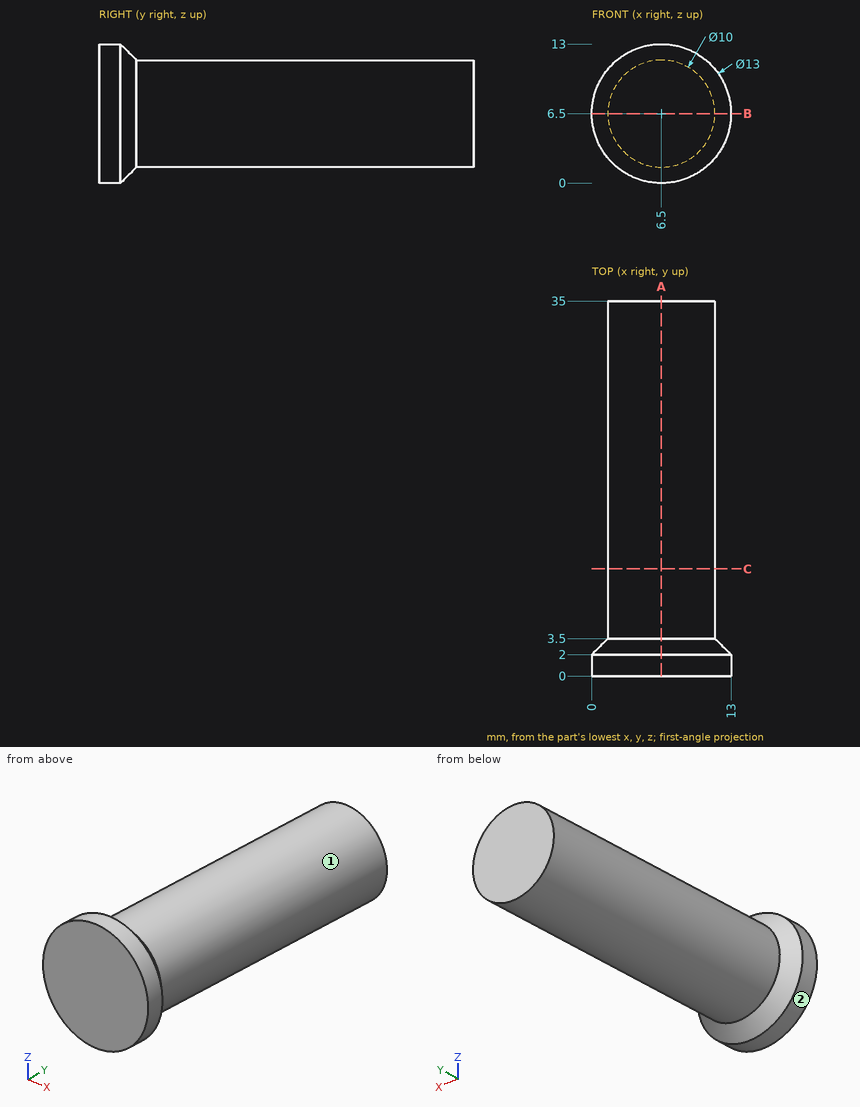
Geometry check sheet. Reference: drawing and pictorial views, mm from the part's lowest x, y, z. A direction names the side the tool comes from. Coordinates: 2 decimals unless noted, no trailing zeros. Write each loop counter-clockwise with the first axis right and the second up, starting at its lowest first coordinate (ties: lowest second). Pieces come first, ordered by that corner, then holes. Notation, with made-up numbers: (46.5, 79) - (95.5, 79) arc R7 ccw to (95.5, 90) - close; hole circle Ø6 at (30, 72). An arc over 180 degrees is marked (long way). Write item = value, one per line.
Q1. Access from +Z, -Z, +X, -X, +Y, -Y to the whole of each face (thin tool, end or side, straight path). Record for the marked faces 1 and 2.
Answer:
face_1 = +Y
face_2 = +Y, -Y
Q2. Material ranges on L1, parallel to X at y = 20, z = 6.25; L2, parallel to Z at x = 9.5, y = 31.5, recorded low to high. Write a range as from..to.
Answer:
L1 = 1.51..11.49
L2 = 2.5..10.5
Q3. Cross-section at B-B (z = 6.5). Enter the section's corners in (x, y).
Answer:
outline = (0, 0) - (13, 0) - (13, 2) - (11.5, 3.5) - (11.5, 35) - (1.5, 35) - (1.5, 3.5) - (0, 2) - close
Q4. Cross-section at A-A (x = 6.5). Enter the section's corners in (y, z), plus the area to 3 significant figures.
Answer:
outline = (0, 0) - (2, 0) - (3.5, 1.5) - (35, 1.5) - (35, 11.5) - (3.5, 11.5) - (2, 13) - (0, 13) - close
area = 358 mm²
Q5. Cross-section at C-C (y = 10). Enter the section's corners in (x, z).
Answer:
outline = circle Ø10 at (6.5, 6.5)
Q6. Go/stop test with flat-tipped pins: pin 1 Ø5 at (y, z) = (12.5, 9) entering from +X; pin 2 Ø6 at (y, z) = (15, 9) entering from -X; pin 3 Ø6 at (x, y) = (2.5, 21.5) entering from +Z. Record where each tip stops, or that it passes through.
Answer:
pin_1 = 11.5
pin_2 = 1.5
pin_3 = 11.4
